Geometry check sheet. Reference: the model listing, model coordinates, mm. A direction names the side the tool comes from. Give positions to 0.01 mm unless a question says otherwise; leave off trailing zeros. Order: outer loops, then holes, each group sorted by start corner. A loop starts at its lowest first (then second) coordinate and runs counter-clockwise, first axis right, second up. Notation, with made-up numbers: M 7,14.25 L 18,14.25 A11 cw 18,21.25 Z; hole C -21.75,87.25 d10. An arc over 180 degrees is marked long. Answer as CSV lines item,"result". Start each with the question number.
Q1. Mould release check, pull along X, two halves, no side actions. Record for faces 1 (the flat face through (14, 5.5, 7)), 2 (the flat face through (-0.9, 2, 0)), 3 (the cylindrical face through (-24.79, -0.89, 10.67)): +X half, -X half, draft (parallel to the pull), parting line (faces both ways), or undercut.
Q2. Go/stop test with flat-tipped pins: pin 1 (2.5 mm diameter, centred on x = 23, y = 1, fed in from +Z) (3 decimals); pin 2 (1.5 mm diameter, centred on x = 14.5, y = 2.5, fed in from +Z); pin 3 (1.6 mm diameter, centred on y = 4, z = 7, fed in from +X); pin 4 (1.9 mm diameter, centred on x = -9, y = 2, fed in from -Z). Record where each tip stops, or that it passes through.
Q3. Thickness scan on line 1 (X direction, y = 1.75, z = 6.25); line 2 (Y direction, x = 16.5, z = -10.25); line 3 (X direction, y = 2.75, z = 0.5). Record the ranges inside material, lowest first.
Q4. Section check C-C, the plane z = 1.5. Record the boundary of the cut face in (x, y).
Q5. Section check D-D, the plane y = 4.5. Record the boundary of the cut face in (x, z).
Q6. Section check B-B, the plane x = 22. Record the boundary of the cut face in (y, z) (3 decimals), then the cut area to 3 significant figures.
Q7. Set-up check for faces 4 (the flat face through (-18.55, 2, 0)), 5 (the flat face through (14, 3, 3.3)), 6 (the flat face through (25.5, -1, 0)), 7 (the flat face through (19.95, 1, 0)): record each of +Z, -Z, +X, -X, +Y, -Y from which the full face is reachable in a straight line by a thin tool's end or side.
Q8. Section check A-A, the plane y = 1.5. Record the boundary of the cut face in (x, z), then the cut area to 3 significant figures.
Autodesk Inventor part; units mm, degrees
ref_plane "YZ Plane" through (0, 0, 0) normal (1, 0, 0) x (0, 1, 0)
ref_plane "XZ Plane" through (0, 0, 0) normal (0, 1, 0) x (-1, 0, 0)
ref_plane "XY Plane" through (0, 0, 0) normal (0, 0, 1) x (1, 0, 0)
sketch "ESP32 Feather" plane through (0, 0, 0) normal (0, 0, 1) x (1, 0, 0)
  line L0 (-25.5, 0) -> (25.5, 0)
  line L1 (25.5, 0) -> (25.5, -1.8)
  line L2 (25.5, -1.8) -> (-25.5, -1.8)
  line L3 (-25.5, -1.8) -> (-25.5, 0)
  line L4 (0, 0) -> (-25.5, 0)
  line L5 (-25.5, 0) -> (-25.5, 0.75)
  line L6 (-25.5, 0.75) -> (0, 0.75)
  line L7 (0, 0.75) -> (0, 0)
  line L8 (-0.9, 0.75) -> (-18.55, 0.75)
  line L9 (-18.55, 0.75) -> (-18.55, 3.1)
  line L10 (-18.55, 3.1) -> (-0.9, 3.1)
  line L11 (-0.9, 3.1) -> (-0.9, 0.75)
  line L12 (10, 0) -> (18, 0)
  line L13 (18, 0) -> (18, 5.5)
  line L14 (18, 5.5) -> (10, 5.5)
  line L15 (10, 5.5) -> (10, 0)
  line L16 (25.6, 0) -> (19.95, 0)
  line L17 (19.95, 0) -> (19.95, 2.45)
  line L18 (19.95, 2.45) -> (25.6, 2.45)
  line L19 (25.6, 2.45) -> (25.6, 0)
  point P0 (0, 0)
  point P1 (0, 0)
  point P2 (-18.55, 0.75)
  point P3 (18, 0)
  point P4 (19.95, 0)
  dimension "d0" = 51
  dimension "d1" = 1.8
  dimension "d2" = 0.75
  dimension "d3" = 25.5
  dimension "d4" = 17.65
  dimension "d5" = 2.35
  dimension "d6" = 24.6
  dimension "d7" = 8
  dimension "d8" = 5.5
  dimension "d9" = 15.5
  dimension "d10" = 2.45
  dimension "d11" = 5.65
  dimension "d25" = 0.1
extrude "PCB" add sketch "ESP32 Feather" along normal mid plane 22.85 contours L0 L1 L2 L3
fillet "Fillet1" radius 2.5 4 edges at (-25.5, -0.9, 11.425) (-25.5, -0.9, -11.425) (25.5, -0.9, -11.425) (25.5, -0.9, 11.425)
extrude "ESP32PCB" add sketch "ESP32 Feather" along normal mid plane 18.1 contours L5 L6 L7 L0
extrude "ESP32Shied" add sketch "ESP32 Feather" along normal mid plane 15.9 contours L9 L10 L11 L6
extrude "Battery Connector" add sketch "ESP32 Feather" along normal blind 11 contours L15 L14 L13 L0
extrude "Extrusion5" cut sketch "ESP32 Feather" along normal blind 3.3 contours L15 L14 L13 L0
extrude "Extrusion6" add sketch "ESP32 Feather" along normal mid plane 8 contours L0 L17 L18 L19 L16
equation "\"d28\" = d26"
equation "\"d29\" = d26"
equation "\"PCB_Width\" = 22.95"
properties part number "ESP32 Feather"
Answer block:
1,face 1,"draft"
1,face 2,"undercut"
1,face 3,"-X half"
2,pin 1,"stops at z = 11.425"
2,pin 2,"stops at z = 11"
2,pin 3,"stops at x = 18"
2,pin 4,"stops at z = -7.95"
3,line 1,"x = -18.55 to -0.9, 10 to 18"
3,line 2,"y = -1.8 to 0"
3,line 3,"x = -18.55 to -0.9"
4,outline,"M -25.5,-1.8 L 25.5,-1.8 L 25.5,0 L 25.6,0 L 25.6,2.45 L 19.95,2.45 L 19.95,0 L 0,0 L 0,0.75 L -0.9,0.75 L -0.9,3.1 L -18.55,3.1 L -18.55,0.75 L -25.5,0.75 Z"
5,outline,"M 10,3.3 L 18,3.3 L 18,11 L 10,11 Z"
6,outline,"M -1.8,-11.425 L 0,-11.425 L 0,-4 L 2.45,-4 L 2.45,4 L 0,4 L 0,11.425 L -1.8,11.425 Z"
6,area,"60.7 mm2"
7,face 4,"+Z, -Z, -X, +Y"
7,face 5,"-Z, +Y"
7,face 6,"+Z, -Z, +X, -Y"
7,face 7,"+Z, -Z, +Y"
8,outline,"M -18.55,-7.95 L -0.9,-7.95 L -0.9,7.95 L -18.55,7.95 Z; M 10,3.3 L 18,3.3 L 18,11 L 10,11 Z; M 19.95,-4 L 25.6,-4 L 25.6,4 L 19.95,4 Z"
8,area,"387 mm2"
